from build123d import *

# Parameters (mm, degrees)
SKETCH_1_R             = 10
EXTRUDE_1_DEPTH        = 300
CUT_EXTRUDE_1_DEPTH    = 3
CHAMFER_1_SIZE         = 0.5
CHAMFER_2_SIZE         = 0.5
PATTERN_LINEAR_1_COUNT = 3
PATTERN_LINEAR_1_PITCH = 120
EXTRUDE_START          = -10
SKETCH_3_R             = 10
EXTRUDE_2_DEPTH        = 110
CHAMFER_3_SIZE         = 1
CUT_EXTRUDE_2_DEPTH    = 60
CUT_EXTRUDE_START      = -20
SKETCH_5_R             = 10
CUT_EXTRUDE_3_DEPTH    = 20
CHAMFER_4_SIZE         = 1


with BuildPart() as part:
    # 草图1 → 凸台-拉伸1 (new body)
    with BuildSketch(Plane(origin=(0, 0, 0), x_dir=(0, 0, -1), z_dir=(1, 0, 0))):
        Circle(SKETCH_1_R)
    extrude(amount=EXTRUDE_1_DEPTH)

    # 草图2 → 切除-拉伸1 (cut)
    with BuildSketch(Plane(origin=(0, 10, 0), x_dir=(1, 0, 0), z_dir=(0, 1, 0))):
        with BuildLine():
            Line((263, 3), (277, 3))
            ThreePointArc((277, 3), (280, 0), (277, -3))
            Line((277, -3), (263, -3))
            ThreePointArc((263, -3), (260, 0), (263, 3))
        make_face()
    cut_extrude_1 = extrude(amount=-CUT_EXTRUDE_1_DEPTH, mode=Mode.SUBTRACT)

    # 倒角1
    chamfer_1_edges = [part.edges().sort_by_distance(p)[0] for p in [
        (0, 0, 10),
    ]]
    chamfer(chamfer_1_edges, length=CHAMFER_1_SIZE)

    # 倒角2
    chamfer_2_edges = [part.edges().sort_by_distance(p)[0] for p in [
        (300, 0, 10),
    ]]
    chamfer(chamfer_2_edges, length=CHAMFER_2_SIZE)

    # 阵列(线性)1: 切除-拉伸1 ×3
    with Locations(*[(-i * PATTERN_LINEAR_1_PITCH, 0, 0) for i in range(1, PATTERN_LINEAR_1_COUNT)]):
        add(cut_extrude_1, mode=Mode.SUBTRACT)

    # 草图3 → 凸台-拉伸2 (add)
    with BuildSketch(Plane(origin=(300, 0, 0), x_dir=(0, 0, -1), z_dir=(1, 0, 0)).offset(EXTRUDE_START)):
        Circle(SKETCH_3_R)
    extrude(amount=EXTRUDE_2_DEPTH)

    # 倒角3
    chamfer_3_edges = [part.edges().sort_by_distance(p)[0] for p in [
        (400, 0, 10),
    ]]
    chamfer(chamfer_3_edges, length=CHAMFER_3_SIZE)

    # 草图4 → 切除-拉伸2 (cut)
    with BuildSketch(Plane(origin=(0, 7, 0), x_dir=(1, 0, 0), z_dir=(0, 1, 0))):
        with BuildLine():
            Line((357, 3), (371, 3))
            ThreePointArc((371, 3), (374, 0), (371, -3))
            Line((371, -3), (357, -3))
            ThreePointArc((357, -3), (354, 0), (357, 3))
        make_face()
    extrude(amount=CUT_EXTRUDE_2_DEPTH, mode=Mode.SUBTRACT)

    # 草图5 → 切除-拉伸3 (cut)
    with BuildSketch(Plane(origin=(400, 0, 0), x_dir=(0, 0, -1), z_dir=(1, 0, 0)).offset(CUT_EXTRUDE_START)):
        Circle(SKETCH_5_R)
    extrude(amount=CUT_EXTRUDE_3_DEPTH, mode=Mode.SUBTRACT)

    # 倒角4
    chamfer_4_edges = [part.edges().sort_by_distance(p)[0] for p in [
        (380, 0, 10),
    ]]
    chamfer(chamfer_4_edges, length=CHAMFER_4_SIZE)


solid = part.part
Here's how the part is built. I have some questions about the finished solid (model axes, mm). A direction names the side the tool comes from. Coordinates: 2 decimals unless noted, no trailing zeros. Order: outer loops, then holes, each group sorted by start corner. A loop starts at its lowest first (then second) coordinate and runs counter-clockwise, first axis right, second up. Notation, with made-up numbers: M -27,75.25 L 21,75.25 A17 ccw 21,93.25 Z; hole C 64.25,24.5 d4. An arc over 180 degrees is marked long. Answer as CSV lines item,"result".
Item 1: For pin 1 (2 mm diameter, centred on x = 33.5, y = 8, fed in from +Z); pin 2 (6.5 mm diameter, centred on x = 154.5, z = -0.5, fed in from +Y); pin 3 (0.8 mm diameter, centred on x = 31.5, y = 8, fed in from -Z), each with a flat end and sliding along its axis, tell me the tip position at first contact or that it passes through.
Results found:
pin 1,"z = 7.14"
pin 2,"y = 9.54"
pin 3,"z = -6.5"
Item 2: We'd pull the mould along X, two halves only. Please class faces 1 (the face through (0, 0, 0)), 2 (the face through (364, 7, 0)), 3 (the face through (380, 0, 0)): +X half, -X half, draft (parallel to the pull), parting line (faces both ways), or undercut.
Results found:
face 1,"-X half"
face 2,"undercut"
face 3,"+X half"
Item 3: On a 3-axis mill with a long thin cutter (end or side, diameter ignored), from which of +Z, -Z, +X, -X, +Y, -Y can I reach the whole of each face in a straight line? I mean faces 4 (the face through (187.1, -9.76, 2.17)), 5 (the face through (270, 7, 0)). Say none if no direction works.
Results found:
face 4,"+X, -X"
face 5,"+Y"
Item 4: Imagine slicing it at A-A on x = 118. Write out the boundary of the cut face in (y, z).
Results found:
outline,"C 0,0 d20"
Item 5: If I drill on line 1 (Z direction, x = 237.5, y = 3.25); line 2 (Z direction, x = 179.5, y = -0.5); line 3 (X direction, y = -4.25, z = -9), over which ranges is the centre line in solid material (lowest first)?
Results found:
line 1,"-9.46 to 9.46"
line 2,"-9.99 to 9.99"
line 3,"0.45 to 379.05"
